Read the model definition and answer for the solid it produces. Units are mm, in the model's axes. A direction names the side the tool comes from. Give positions to 0.01 mm unless a question says otherwise; leave off trailing zeros. Write each loop counter-clockwise with the first axis right and the second up, starting at its lowest first coordinate (ties: lowest second). Pieces come first, ordered by that corner, then holes. Notation, with made-up numbers: (12.25, -14.5) -> (47.25, -14.5) arc R13 ccw to (47.25, 3.5) -> close; hole circle Ø11 at (-30, 45). An arc over 180 degrees is marked (long way). Use a Markdown table: item, result.
from build123d import *

# Parameters (mm, degrees)
BOSS_EXTRUDE1_DEPTH = 12
SKETCH2_W           = 58
SKETCH2_H           = 28.2
BOSS_EXTRUDE2_DEPTH = 2
SHELL2_START        = 2
SHELL2_DEPTH        = 10
SKETCH3_R           = 11
SKETCH3_R_2         = 1.25
CUT_EXTRUDE1_DEPTH  = 2
FILLET1_R           = 2
SKETCH4_R           = 1.7
CUT_EXTRUDE2_DEPTH  = 2
SKETCH5_R           = 1.7
CUT_EXTRUDE3_DEPTH  = 2
SKETCH7_R           = 1.25
CUT_EXTRUDE6_DEPTH  = 14
SKETCH8_R           = 1.25
CUT_EXTRUDE7_DEPTH  = 17


# Read off the part's stored shape, not the designer's step: Shell2
with BuildPart() as part:
    # Sketch1 → Boss-Extrude1 (new body)
    with BuildSketch(Plane.XY):
        with BuildLine():
            Line((0, 14), (0, -14))
            ThreePointArc((0, -14), (14, 0), (0, 14))
        make_face()
    extrude(amount=BOSS_EXTRUDE1_DEPTH)

    # Sketch2 → Boss-Extrude2 (add)
    with BuildSketch(Plane.XY.offset(12)):
        with Locations((4.15, 0)):
            Rectangle(SKETCH2_W, SKETCH2_H)
    extrude(amount=BOSS_EXTRUDE2_DEPTH)

    # Shell2 outline → Shell2 (cut)
    with BuildSketch(Plane.XY.offset(SHELL2_START)):
        with BuildLine():
            ThreePointArc((0, -12), (12, 0), (0, 12))
            Line((0, 12), (0, -12))
        make_face()
    extrude(amount=SHELL2_DEPTH, mode=Mode.SUBTRACT)

    # Sketch3 → Cut-Extrude1 (cut)
    with BuildSketch(Plane.XY.offset(14)):
        with Locations((-10.75, 0)):
            Circle(SKETCH3_R)
        with Locations((-22.25, 11.5)):
            Circle(SKETCH3_R_2)
        with Locations((-22.25, -11.5)):
            Circle(SKETCH3_R_2)
        with Locations(Location((0.75, -11.5, 0), (0, 0, 344.215225354))):
            Circle(SKETCH3_R_2)
        with Locations(Location((0.75, 11.5, 0), (0, 0, 15.784774646))):
            Circle(SKETCH3_R_2)
    extrude(amount=-CUT_EXTRUDE1_DEPTH, mode=Mode.SUBTRACT)

    # Fillet1
    fillet1_edges = [part.edges().sort_by_distance(p)[0] for p in [
        (-24.85, 14.1, 13),
        (-24.85, -14.1, 13),
        (33.15, -14.1, 13),
        (33.15, 14.1, 13),
    ]]
    fillet(fillet1_edges, radius=FILLET1_R)

    # Sketch4 → Cut-Extrude2 (cut)
    with BuildSketch(Plane.XY.offset(14)):
        with Locations((26.15, 8)):
            Circle(SKETCH4_R)
        with Locations((26.15, -8)):
            Circle(SKETCH4_R)
        with Locations((8.65, 0)):
            Circle(SKETCH4_R)
    extrude(amount=-CUT_EXTRUDE2_DEPTH, mode=Mode.SUBTRACT)

    # Sketch5 → Cut-Extrude3 (cut)
    with BuildSketch(Plane(origin=(0, 0, 0), x_dir=(-1, 0, 0), z_dir=(0, 0, -1))):
        with Locations((-5, -9)):
            Circle(SKETCH5_R)
        with Locations((-5, 9)):
            Circle(SKETCH5_R)
    extrude(amount=-CUT_EXTRUDE3_DEPTH, mode=Mode.SUBTRACT)

    # Sketch7 → Cut-Extrude6 (cut)
    with BuildSketch(Plane(origin=(0, 0, 0), x_dir=(0, 0, -1), z_dir=(1, 0, 0))):
        with Locations(Location((-5, 0, 0), (0, 0, 180))):
            Circle(SKETCH7_R)
    extrude(amount=CUT_EXTRUDE6_DEPTH, mode=Mode.SUBTRACT)

    # Sketch8 → Cut-Extrude7 (cut, symmetric)
    with BuildSketch(Plane(origin=(0, 0, 0), x_dir=(1, 0, 0), z_dir=(0, 1, 0))):
        with Locations(Location((2.5, -5, 0), (0, 0, 270))):
            Circle(SKETCH8_R)
    extrude(amount=CUT_EXTRUDE7_DEPTH, both=True, mode=Mode.SUBTRACT)


solid = part.part
Item 1: A cutting plane is placed at C-C (y = 5.5). Give the vertices of the cut face in (x, z).
Return value:
| item | result |
|---|---|
| outline | (-24.85, 12) -> (-20.28, 12) -> (-20.28, 14) -> (-24.85, 14) -> close; (-1.22, 12) -> (10.67, 12) -> (10.67, 2) -> (0, 2) -> (0, 0) -> (12.87, 0) -> (12.87, 12) -> (33.15, 12) -> (33.15, 14) -> (-1.22, 14) -> close |
Item 2: Each of these flat-tipped pins is pushed along its axis until it touches: P1, Ø6, axis at x = -10.5, z = 10.5, coming from the +Y side; P2, Ø3, axis at x = -22.25, y = -11.5, coming from the -Z side; P3, Ø1.5, axis at y = -4.5, z = 9.5, coming from the +X side; P4, Ø3, axis at x = 2.5, z = 5, coming from the -Y side. Where does it stop, or does it pass through?
Return value:
| item | result |
|---|---|
| P1 | y = 14.1 |
| P2 | z = 12 |
| P3 | x = 13.49 |
| P4 | y = -13.96 |
Item 3: A cutting plane is placed at B-B (x = 26.15). Give the vertices of the cut face in (y, z).
Return value:
| item | result |
|---|---|
| outline | (-14.1, 12) -> (-9.7, 12) -> (-9.7, 14) -> (-14.1, 14) -> close; (-6.3, 12) -> (6.3, 12) -> (6.3, 14) -> (-6.3, 14) -> close; (9.7, 12) -> (14.1, 12) -> (14.1, 14) -> (9.7, 14) -> close |
Item 4: A cutting plane is placed at A-A (x = 5). Give the vertices of the cut face in (y, z), then the cut area to 3 significant figures.
Return value:
| item | result |
|---|---|
| outline | (-14.1, 12) -> (-13.08, 12) -> (-13.08, 0) -> (-10.7, 0) -> (-10.7, 2) -> (-10.91, 2) -> (-10.91, 12) -> (10.91, 12) -> (10.91, 2) -> (10.7, 2) -> (10.7, 0) -> (13.08, 0) -> (13.08, 12) -> (14.1, 12) -> (14.1, 14) -> (-14.1, 14) -> close; (-7.3, 0) -> (7.3, 0) -> (7.3, 2) -> (-7.3, 2) -> close |
| area | 138 mm^2 |
Item 5: A cutting plane is placed at D-D (z = 12.75). Count the separate pieces of the cut face and the enclosed holes in it, then the cut area to 3 significant figures.
Return value:
| item | result |
|---|---|
| separate pieces | 1 |
| enclosed holes | 8 |
| area | 1,210 mm^2 |
Item 6: For a pull along Y with two mould halves and no side action, classify faces 1 (the face through (-21.578, 12.554, 13.014)), 2 (the face through (0, 0, 1)), 3 (the face through (4, 14.1, 13)) as +Y half, -Y half, draft (parallel to the pull), parting line (faces both ways), or undercut.
Return value:
| item | result |
|---|---|
| face 1 | undercut |
| face 2 | draft |
| face 3 | +Y half |
Item 7: Straight lines are drawn through the part: line 1 along Y through (x, z) = (26.15, 13.35); line 2 along Y through (x, z) = (-22, 12.75); line 3 along Z through (x, y) = (10.5, 1). For each, find the intervals that lie inside material, in ascending order. Write a range as [from, to].
Return value:
| item | result |
|---|---|
| line 1 | [-14.1, -9.7], [-6.3, 6.3], [9.7, 14.1] |
| line 2 | [-14.1, -12.72], [-10.28, 10.28], [12.72, 14.1] |
| line 3 | [0, 2], [12, 14] |
Item 8: A tool of negligible diameter and unlimited length cuts with its end or side. For faces 4 (the face through (12, 0, 7)), 5 (the face through (5.37, 7.34, 0.99)), 6 (the face through (6.95, 0.07, 13.01)), 7 (the face through (10, -3, 12)), 8 (the face through (-24.28, -13.5, 13.01)), from which of +Z, -Z, +X, -X, +Y, -Y can it reach the whole face along a straight path? Write none if from no direction.
Return value:
| item | result |
|---|---|
| face 4 | -X |
| face 5 | -Z |
| face 6 | +Z |
| face 7 | none |
| face 8 | +Z, -Z, -X, -Y |
